Autodesk Inventor part; units mm, degrees
ref_plane "YZ Plane" through (0, 0, 0) normal (1, 0, 0) x (0, 1, 0)
ref_plane "XZ Plane" through (0, 0, 0) normal (0, 1, 0) x (-1, 0, 0)
ref_plane "XY Plane" through (0, 0, 0) normal (0, 0, 1) x (1, 0, 0)
sketch "Esboço4" plane through (0, 0, 0) normal (0, 1, 0) x (-1, 0, 0)
  line L0 (0, -15) -> (0, -135)
  line L1 (-15, -150) -> (-55, -150)
  line L2 (-70, -135) -> (-70, -15)
  line L3 (-55, 0) -> (-15, 0)
  arc A0 (-15, -150) -> (0, -135) centre (-15, -135) ccw
  arc A1 (-70, -135) -> (-55, -150) centre (-55, -135) ccw
  arc A2 (-55, 0) -> (-70, -15) centre (-55, -15) ccw
  arc A3 (0, -15) -> (-15, 0) centre (-15, -15) ccw
  point P0 (0, 0)
  point P1 (0, -150)
  point P2 (-70, -150)
  dimension "d7" = 150
  dimension "d8" = 70
  dimension "d9" = 15
extrude "Extrusão2" add sketch "Esboço4" along normal blind 5
sketch "Esboço5" plane through (0, 5, 0) normal (0, 1, 0) x (1, 0, 0)
  line L0 (15, 0) -> (55, 0)
  line L1 (55, 150) -> (15, 150)
  circle A0 centre (35, 61) radius 2.5
  circle A1 centre (35, 68) radius 2.5
  point P0 (0, 0)
extrude "Extrusão3" cut sketch "Esboço5" against normal through all
sketch "Sketch7" plane through (0, 0, 0) normal (0, -1, 0) x (1, 0, 0)
  circle A0 centre (35, -61) radius 2
  circle A1 centre (35, -68) radius 2
  line L0 (43, -68) -> (43, -74.75)
  line L1 (43, -74.75) -> (27, -74.75)
  line L2 (27, -74.75) -> (27, -54.25)
  line L3 (27, -54.25) -> (43, -54.25)
  line L4 (43, -54.25) -> (43, -68)
  point P0 (0, 0)
  dimension "d25" = 8
extrude "Extrusion4" add sketch "Sketch7" along normal blind 6
fillet "Fillet4" radius 2 8 edges at (43, -3, -54.25) (43, -3, -74.75) (43, -6, -64.5) (35, -6, -54.25) (27, -6, -64.5) (35, -6, -74.75) (27, -3, -74.75) (27, -3, -54.25)
fillet "Fillet5" radius 0.5 2 edges at (32.5, 5, -61) (32.5, 5, -68)
fillet "Fillet7" radius 2 8 edges at (65.6066, 0, -145.6066) (35, 0, -150) (4.3934, 0, -145.6066) (0, 0, -75) (4.3934, 0, -4.3934) (35, 0, 0) (65.6066, 0, -4.3934) (70, 0, -75)
properties part number "Base superior(suporte)_3DPrint"
For this review, take the finished solid that the model builds, in its own axes (mm). A direction names the side the tool comes from. Round coordinates to 2 decimals unless told otherwise and drop trailing zeros. Order: outer loops, then holes, each group sorted by start corner. A loop starts at its lowest first (then second) coordinate and runs counter-clockwise, first axis right, second up. Notation, with made-up numbers: (2.5, -39) -> (38.5, -39) arc R23 ccw to (38.5, -10) -> close; hole circle Ø7 at (0.5, -37.75). An arc over 180 degrees is marked (long way). Write item = value, one per line. Start each with the question number.
1) Insertion check: pin 1 (3 mm diameter, centred on x = 33, y = -2, fed in from -Z); pin 2 (6 mm diameter, centred on x = 57, y = 0, fed in from -Z); pin 3 (2 mm diameter, centred on y = -2.5, z = -63, fed in from +X); pin 4 (2.5 mm diameter, centred on x = 35, z = -68, fed in from +Y). Each pin has a flat end and moves straight along its axis. Give the tip position at first contact, or say it passes through.
2) Take a section at A-A on z = -68. State the section outline as (x, y) points.
3) Take a section at D-D on x = 45. State the section outline as (y, z) points, plus the area to 3 significant figures.
4) Take a section at B-B on y = -1.5. State the section outline as (x, z) points.
5) The part is to be moulded in two halves that separate along Z. For faces 1 (the face through (43, 0, -74)), 2 (the face through (35, -2, -54.25)), 3 (the face through (37.31, 2.28, -67.04)), say which applies: +Z half, -Z half, draft (parallel to the pull), parting line (faces both ways), or undercut.
6) Tool access review of faces 4 (the face through (35, -2, -74.75)), 5 (the face through (43, -2, -64)), 6 (the face through (27, -2, -65)), 7 (the face through (34, 0, -59)), 8 (the face through (35, -3, -63)): name each direction out of +Z, -Z, +X, -X, +Y, -Y from which nothing blocks a thin tool from reaching the whole face with its end or side.
7) To check wall thickness, follow line 1 (Z direction, x = 35, y = -4.1); line 2 (Z direction, x = 35, y = 2.4); line 3 (Y direction, x = 57, z = -20). State the ranges of each line that lie inside material, in increasing order. Write a range as from..to.
8) Take a section at C-C on x = 35. Count the separate pieces of the cut face and the enclosed holes in it, plus the area to 3 significant figures.
Verdict:
q1.pin_1 = -74.75
q1.pin_2 = -150
q1.pin_3 = 43
q1.pin_4 = through
q2.outline = (0, 2) arc R2 ccw to (2, 0) -> (27, 0) -> (27, -4) arc R2 ccw to (29, -6) -> (33, -6) -> (33, 0) -> (32.5, 0) -> (32.5, 4.5) arc R0.5 ccw to (32, 5) -> (0, 5) -> close; (37, -6) -> (41, -6) arc R2 ccw to (43, -4) -> (43, 0) -> (68, 0) arc R2 ccw to (70, 2) -> (70, 5) -> (38, 5) arc R0.5 ccw to (37.5, 4.5) -> (37.5, 0) -> (37, 0) -> close
q3.outline = (0, -148) arc R2 ccw to (2, -150) -> (5, -150) -> (5, 0) -> (2, 0) arc R2 ccw to (0, -2) -> close
q3.area = 748 mm2
q4.outline = (27, -72.75) arc R2 ccw to (29, -74.75) -> (41, -74.75) arc R2 ccw to (43, -72.75) -> (43, -56.25) arc R2 ccw to (41, -54.25) -> (29, -54.25) arc R2 ccw to (27, -56.25) -> close; hole circle Ø4 at (35, -68); hole circle Ø4 at (35, -61)
q5.face_1 = draft
q5.face_2 = +Z half
q5.face_3 = undercut
q6.face_4 = -Z, +X, -X, -Y
q6.face_5 = +Z, -Z, +X, -Y
q6.face_6 = +Z, -Z, -X, -Y
q6.face_7 = +Y
q6.face_8 = +Y, -Y
q7.line_1 = -74.75..-70, -66..-63, -59..-54.25
q7.line_2 = -150..-70.5, -65.5..-63.5, -58.5..0
q7.line_3 = 0..5
q8.separate_pieces = 3
q8.enclosed_holes = 0
q8.area = 771 mm2
